```python
from build123d import *

# Parameters (mm, degrees)
SKETCH1_R           = 3.1
BOSS_EXTRUDE1_DEPTH = 9
SKETCH3_R           = 2
CUT_EXTRUDE1_DEPTH  = 10


with BuildPart() as part:
    # Sketch1 → Boss-Extrude1 (new, symmetric)
    with BuildSketch(Plane.XY):
        Polygon((-35, 0), (35, 0), (35, 45), (11, 45), (-35, 20), align=None)
        with Locations((21, 30)):
            Circle(SKETCH1_R, mode=Mode.SUBTRACT)
    extrude(amount=BOSS_EXTRUDE1_DEPTH, both=True)

    # Sketch3 → Cut-Extrude1 (cut)
    with BuildSketch(Plane.XZ):
        with Locations(Location((19, -5.5, 0), (0, 0, 270))):
            Circle(SKETCH3_R)
        with Locations(Location((-13, -5.5, 0), (0, 0, 270))):
            Circle(SKETCH3_R)
    extrude(amount=-CUT_EXTRUDE1_DEPTH, mode=Mode.SUBTRACT)


solid = part.part
```
Source: CAD feature listing. Evaluate the final solid. Frame: model axes, mm. A direction names the side the tool comes from. Coordinates: 2 decimals unless noted, no trailing zeros. Order: outer loops, then holes, each group sorted by start corner. A loop starts at its lowest first (then second) coordinate and runs counter-clockwise, first axis right, second up. Notation, with made-up numbers: M 71.25,-18.5 L 86.25,-18.5 A16 cw 86.25,7.5 Z; hole C 14,-20 d11. An arc over 180 degrees is marked long. Write each question's results on one line, items separated by ' | '. Start each with the question number.
1) Contact query for flat-ended pins moving along their axis: pin 1 Ø2 at (x, z) = (-13.5, -6) entering from -Y; pin 2 Ø5 at (y, z) = (33.5, 6.5) entering from -X. Output: stop coordinate, or through.
2) Section query A-A (y = 30). Return the cut outline in (x, z).
3) Section query D-D (x = -13). Return the cut outline in (y, z), plus the area to 3 significant figures.
4) Access query for faces 5 (the face through (20.596, 33.074, -0.126)), 6 (the face through (-13, 10, -5)). Directions: +Z, -Z, +X, -X, +Y, -Y. A direction counts if a zero-diameter tool reaches every point of the face in a straight line with its end or side. Return the directions, or none.
5) Draft query along Z for faces 1 (the face through (20.983, 4.93, -5.24)), 2 (the face through (-11.678, 32.675, 0.126)), 3 (the face through (19, 10, -5)), 4 (the face through (7, 18, 9)). Return one class per face: released by +Z, released by -Z, zero draft, split by the parting line, or undercut.
6) Section query B-B (z = 1). Return the cut outline in (x, y).
7) Section query C-C (x = 19). Return the cut outline in (y, z), plus the area to 3 significant figures.
8) Line query: line 1 (X direction, y = 8, z = -5.5); line 2 (Y direction, x = 21, z = 1.5); line 3 (X direction, y = 7, z = -7). Output: solid intervals per line, ascending. Write a range as from..to.
Answers:
1) pin 1: stops at y = 10 | pin 2: stops at x = -14.76
2) outline: M -16.6,-9 L 17.9,-9 L 17.9,9 L -16.6,9 Z; M 24.1,-9 L 35,-9 L 35,9 L 24.1,9 Z
3) outline: M 0,-9 L 31.96,-9 L 31.96,9 L 0,9 L 0,-3.5 L 10,-3.5 L 10,-7.5 L 0,-7.5 Z | area: 535 mm^2
4) face 5: +Z, -Z | face 6: -Y
5) face 1: undercut | face 2: zero draft | face 3: undercut | face 4: released by +Z
6) outline: M -35,0 L 35,0 L 35,45 L 11,45 L -35,20 Z; hole C 21,30 d6.2
7) outline: M 0,-9 L 27.63,-9 L 27.63,9 L 0,9 L 0,-3.5 L 10,-3.5 L 10,-7.5 L 0,-7.5 Z; M 32.37,-9 L 45,-9 L 45,9 L 32.37,9 Z | area: 685 mm^2
8) line 1: x = -35..-15, -11..17, 21..35 | line 2: y = 0..26.9, 33.1..45 | line 3: x = -35..-14.32, -11.68..17.68, 20.32..35
